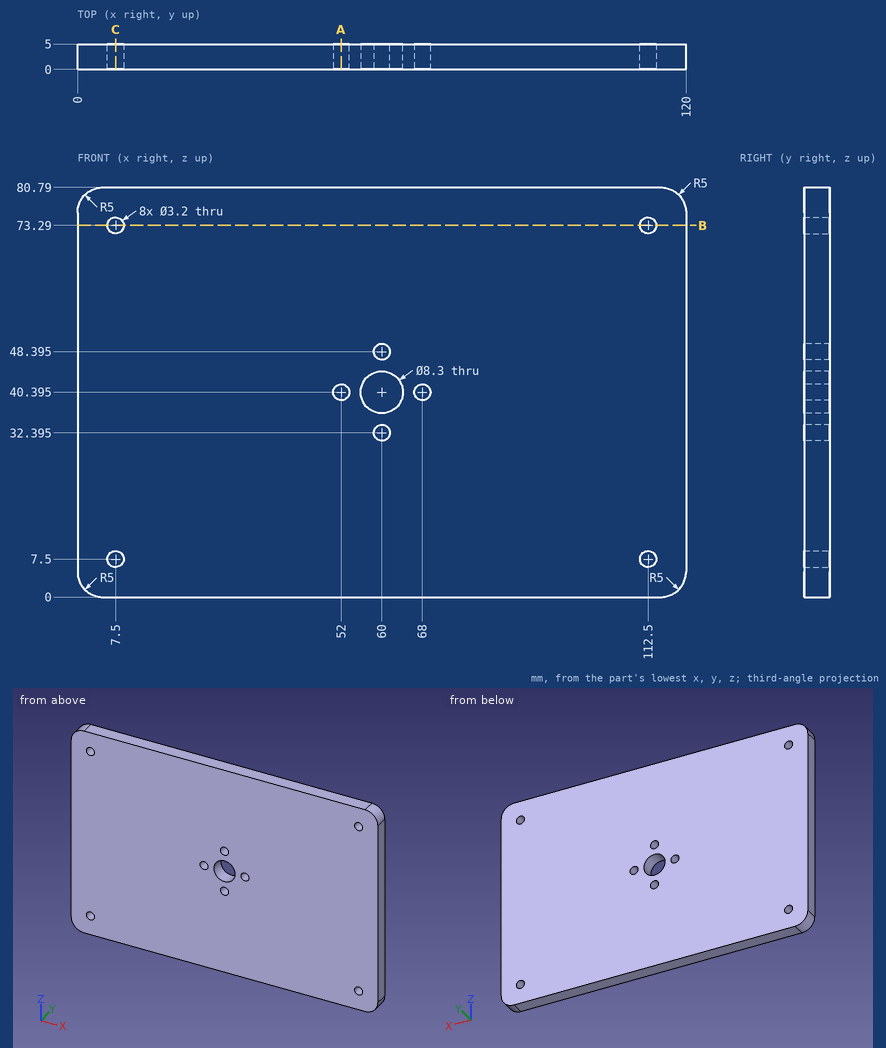
Here's the drawing with two shaded views (mm, measured from the low corner). I have some questions. Coordinates: 2 decimals unless noted, no trailing zeros. Loops run counter-clockwise (first coordinate to the right, second up) from the corner with the lowest first, then second, coordinate; pieces in that order, holes last. Notation, with made-up numbers: M 50.25,63.5 L 87.25,63.5 A23 cw 87.25,98.5 Z; hole C 28,61.25 d10. An arc over 180 degrees is marked long. Return JSON: item names as keys, results as strings. Group by question number.
Item 1: Imagine slicing it at C-C (x = 7.5). Please give me the cut outline in (y, z), and give its area (3 significant figures).
Item 2: Imagine slicing it at A-A (x = 52). Please give me the cut outline in (y, z) (3 decimals).
Item 3: Imagine slicing it at B-B (z = 73.29). Please give me the cut outline in (x, y), and give its area (3 significant figures).
Item 4: If I drill on L1, parallel to Z at x = 60, y = 1.9 (3 decimals); L2, parallel to Z at x = 112.5, y = 1.2; L3, parallel to X at y = 3.1, z = 7.5, over which ranges is the centre line in solid material (lowest first)? Write a range as from..to.
Verdict:
{
 "1": {"outline": "M 0,0 L 5,0 L 5,5.9 L 0,5.9 Z; M 0,9.1 L 5,9.1 L 5,71.69 L 0,71.69 Z; M 0,74.89 L 5,74.89 L 5,80.79 L 0,80.79 Z", "area": "372 mm^2"},
 "2": {"outline": "M 0,0 L 5,0 L 5,38.795 L 0,38.795 Z; M 0,41.995 L 5,41.995 L 5,80.79 L 0,80.79 Z"},
 "3": {"outline": "M 0,0 L 5.9,0 L 5.9,5 L 0,5 Z; M 9.1,0 L 110.9,0 L 110.9,5 L 9.1,5 Z; M 114.1,0 L 120,0 L 120,5 L 114.1,5 Z", "area": "568 mm^2"},
 "4": {"L1": "z = 0..30.795, 33.995..36.245, 44.545..46.795, 49.995..80.79", "L2": "z = 0..5.9, 9.1..71.69, 74.89..80.79", "L3": "x = 0..5.9, 9.1..110.9, 114.1..120"}
}
